Geometry check sheet. Reference: the model listing, model coordinates, mm. A direction names the side the tool comes from. Give positions to 0.01 mm unless a question says otherwise; leave off trailing zeros. Order: outer loops, then holes, each group sorted by start corner. A loop starts at its lowest first (then second) coordinate and runs counter-clockwise, first axis right, second up. Notation, with made-up numbers: M 11,73.25 L 46,73.25 A24 cw 46,104.25 Z; hole C 9.5,-5 d10. An arc over 180 degrees is marked long. Answer as CSV lines item,"result".
from build123d import *

# Parameters (mm, degrees)
F0_W     = 80
F0_H     = 80
F1_DEPTH = 10
F2_W     = 4
F2_H     = 4
F3_DEPTH = 2


with BuildPart() as f1:
    # F0 (on Top) → F1 (new body)
    with BuildSketch(Plane.XY):
        Rectangle(F0_W, F0_H)
    extrude(amount=F1_DEPTH)

    # F2 (on Front) → F3 (join, symmetric)
    with BuildSketch(Plane.XZ):
        with Locations((26, 12)):
            Rectangle(F2_W, F2_H)
        with Locations((34, 12)):
            Rectangle(F2_W, F2_H)
    extrude(amount=F3_DEPTH, both=True)


solid = f1.part
(1) Section check A-A on z = 12.5. Enter the section's corners in (x, y), then the cut area to 3 significant figures.
The answers:
outline,"M 24,-2 L 28,-2 L 28,2 L 24,2 Z; M 32,-2 L 36,-2 L 36,2 L 32,2 Z"
area,"32.0 mm2"
(2) Section check C-C on x = -9.5. Enter the section's corners in (y, z), then the cut area to 3 significant figures.
The answers:
outline,"M -40,0 L 40,0 L 40,10 L -40,10 Z"
area,"800 mm2"
(3) Draft check along X on faces 4 (the face through (36, 0, 12)), 5 (the face through (28, 0, 12)), 6 (the face through (34, 2, 12)). Enter one of: +X half, -X half, draft (parallel to the pull), parting line (faces both ways), or undercut.
The answers:
face 4,"+X half"
face 5,"undercut"
face 6,"draft"
(4) Tool access check on faces 1 (the face through (34, -2, 12)), 2 (the face through (32, 0, 12)), 3 (the face through (24, 0, 12)). Record the directions out of +Z, -Z, +X, -X, +Y, -Y that give a thin tool (end or side, any length) a straight path to the whole face; none if there is none.
The answers:
face 1,"+Z, +X, -X, -Y"
face 2,"+Z, +Y, -Y"
face 3,"+Z, -X, +Y, -Y"
(5) Material ranges on line 1 (Z direction, x = 15.5, y = 22); line 2 (Y direction, x = 32.5, z = 13.25), recorded low to high.
The answers:
line 1,"z = 0 to 10"
line 2,"y = -2 to 2"
(6) Gauge pin test, flat ends, axial feed: P1, Ø2, axis at y = -0.5, z = 12.5, coming from the -X side; P2, Ø3, axis at x = 25.5, z = 13, coming from the +Y side; P3, Ø3, axis at y = 0.5, z = 13, coming from the +X side. Record the tip position at first contact, or that the pin passes through.
The answers:
P1,"stops at x = 24"
P2,"stops at y = 2"
P3,"stops at x = 36"
(7) Section check B-B on y = 1. Enter the section's corners in (x, z).
The answers:
outline,"M -40,0 L 40,0 L 40,10 L 36,10 L 36,14 L 32,14 L 32,10 L 28,10 L 28,14 L 24,14 L 24,10 L -40,10 Z"
